Source: CAD feature listing. Evaluate the final solid. Frame: model axes, mm. A direction names the side the tool comes from. Round coordinates to 2 decimals unless told otherwise and drop trailing zeros. Write each loop counter-clockwise with the first axis right and the second up, starting at its lowest first coordinate (ties: lowest second). Pieces come first, ordered by that corner, then holes. Notation, with made-up numbers: M 61.25,85 L 105.25,85 A11 cw 105.25,99 Z; hole C 59,-35 d7. An arc over 180 degrees is marked long. Answer in a Markdown table with one row per item. Add a question column.
Item 1: Cut plane A-A on z = 0. Return loops of the section in (x, y), and give its area (3 significant figures).
Item 2: Set-up query: faces 4 (the face through (1.48, -10.25, -0.05)), 5 (the face through (1, -3, 6)), 6 (the face through (1, -3, -6)), 7 (the face through (1, 6, -3)), 8 (the face through (1, 3, 6)). Return all of +Z, -Z, +X, -X, +Y, -Y with unobstructed straight access to the full face (end or side cutting, diameter ignored); none if empty.
Item 3: Cut plane D-D on z = 6.25. Return loops of the section in (x, y).
Item 4: Cut plane B-B on y = 2.75. Return loops of the section in (x, z), and give its area (3 significant figures).
Item 5: Contact query for flat-ended pins moving along their axis: pin 1 (1.5 mm diameter, centred on x = 2, y = 6.5, fed in from -Z); pin 2 (1 mm diameter, centred on x = 1.5, z = -6.5, fed in from -Y); pin 3 (1 mm diameter, centred on x = 1, y = -5.5, fed in from +Z); pin 4 (2 mm diameter, centred on y = 9, z = 0, fed in from -X). Output: stop coordinate, or through.
Item 6: Mould query, pull axis Z, two halves, no side actions, for faces 1 (the face through (1, -2, -4)), 2 (the face through (1, 6, 3)), 3 (the face through (0, 0, 0)). Classes: released by +Z, released by -Z, zero draft, split by the parting line, or undercut.
Item 7: Cut plane C-C on x = 0.3. Return loops of the section in (y, z), and give its area (3 significant figures).
Item 8: Material intervals for probe 1 along Z at (x, y) = (1.25, -9); probe 2 along Z at (x, y) = (2, -3.5), sorted ascending.
Autodesk Inventor part; units mm, degrees
ref_plane "YZ Plane" through (0, 0, 0) normal (1, 0, 0) x (0, 1, 0)
ref_plane "XZ Plane" through (0, 0, 0) normal (0, 1, 0) x (-1, 0, 0)
ref_plane "XY Plane" through (0, 0, 0) normal (0, 0, 1) x (1, 0, 0)
sketch "スケッチ1" plane through (0, 0, 0) normal (1, 0, 0) x (0, 1, 0)
  line L0 (9, 0) -> (-9, 0) construction
  line L1 (9, 3) -> (-9, 3)
  line L2 (-9, -3) -> (9, -3)
  arc A0 (9, -3) -> (9, 3) centre (9, 0) ccw
  arc A1 (-9, 3) -> (-9, -3) centre (-9, 0) ccw
  line L3 (3, 7) -> (-3, 7)
  line L4 (-3, -7) -> (3, -7)
  line L5 (3, 7) -> (-3, -7) construction
  line L6 (-3, 7) -> (3, -7) construction
  arc A2 (3, 5) -> (3, 3) centre (3, 4) ccw
  arc A3 (-3, 3) -> (-3, 5) centre (-3, 4) ccw
  arc A4 (-3, -5) -> (-3, -3) centre (-3, -4) ccw
  arc A5 (3, -3) -> (3, -5) centre (3, -4) ccw
  line L7 (-3, 7) -> (-3, 5)
  line L8 (3, 5) -> (3, 7)
  line L9 (3, -7) -> (3, -5)
  line L10 (3, -3) -> (3, 3)
  line L11 (-3, 3) -> (-3, -3)
  line L12 (-3, -5) -> (-3, -7)
  circle A6 centre (-9, 0) radius 1.25
  circle A7 centre (9, 0) radius 1.25
  point P0 (0, 0)
  dimension "d0" = 6
  dimension "d1" = 6
  dimension "d2" = 1
  dimension "d3" = 14
  dimension "d4" = 18
  dimension "d7" = 0
  dimension "d8" = 6
  dimension "d9" = 4
  dimension "d10" = 6
  dimension "d11" = 2.5
  dimension "d12" = 2.5
extrude "押し出し1" add sketch "スケッチ1" along normal blind 3
properties part number "tip" material "アルミニウム 2014-T4"
Results below:
| question | item | result |
|---|---|---|
| 1 | outline | M 0,-12 L 3,-12 L 3,-10.25 L 0,-10.25 Z; M 0,-7.75 L 3,-7.75 L 3,7.75 L 0,7.75 Z; M 0,10.25 L 3,10.25 L 3,12 L 0,12 Z |
| 1 | area | 57.0 mm2 |
| 2 | face 4 | +X, -X |
| 2 | face 5 | +Z, +X, -X, -Y |
| 2 | face 6 | -Z, +X, -X, -Y |
| 2 | face 7 | -Z, +X, -X, +Y |
| 2 | face 8 | +Z, +X, -X, +Y |
| 3 | outline | M 0,-3 L 3,-3 L 3,3 L 0,3 Z |
| 4 | outline | M 0,-7 L 3,-7 L 3,-4.97 L 0,-4.97 Z; M 0,-3.03 L 3,-3.03 L 3,3.03 L 0,3.03 Z; M 0,4.97 L 3,4.97 L 3,7 L 0,7 Z |
| 4 | area | 30.4 mm2 |
| 5 | pin 1 | z = -3 |
| 5 | pin 2 | y = -3 |
| 5 | pin 3 | z = 3 |
| 5 | pin 4 | through |
| 6 | face 1 | undercut |
| 6 | face 2 | released by +Z |
| 6 | face 3 | zero draft |
| 7 | outline | M -9,-3 L -3,-3 A1 cw -3,-5 L -3,-7 L 3,-7 L 3,-5 A1 cw 3,-3 L 9,-3 A3 ccw 9,3 L 3,3 A1 cw 3,5 L 3,7 L -3,7 L -3,5 A1 cw -3,3 L -9,3 A3 ccw Z; hole C -9,0 d2.5; hole C 9,0 d2.5 |
| 7 | area | 168 mm2 |
| 8 | probe 1 | -3 to -1.25, 1.25 to 3 |
| 8 | probe 2 | -3 to 3 |
